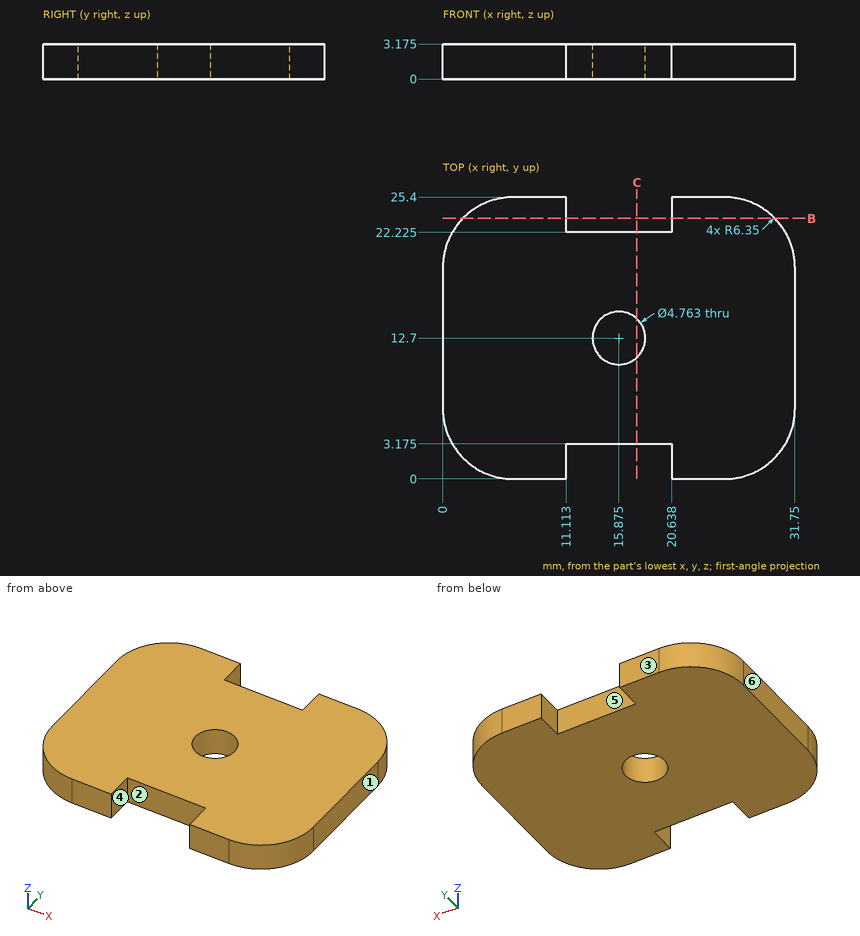
For this review, use the dimensioned drawing (mm, ordinates from the lowest corner) and the shaded views. A direction names the side the tool comes from. Coordinates: 2 decimals unless noted, no trailing zeros. Order: outer loops, then holes, each group sorted by start corner. A loop starts at its lowest first (then second) coordinate and runs counter-clockwise, first axis right, second up. Notation, with made-up numbers: (51, 45) - (67, 45) arc R18 ccw to (67, 50) - close; hole circle Ø1 at (-8, -29). An arc over 180 degrees is marked (long way). Answer in a Markdown table with one row per item.
(1) Consider section C-C on x = 17.5. State the section outline as (y, z) points (1 decimal).
Checked values:
| item | result |
|---|---|
| outline | (3.2, 0) - (11, 0) - (11, 3.2) - (3.2, 3.2) - close; (14.4, 0) - (22.2, 0) - (22.2, 3.2) - (14.4, 3.2) - close |
(2) Clearance check with flat-ended pins moving along their axes: pin 1 (1 mm diameter, centred on y = 1, z = 2, fed in from -X); pin 2 (7.5 mm diameter, centred on x = 15.875, y = 12.7, fed in from -Z); pin 3 (1.6 mm diameter, centred on y = 23, z = 2, fed in from +X) (1 decimal); pin 4 (1 mm diameter, centred on x = 16, z = 2, fed in from +Y) (1 decimal). State where each tip first meets the part, or that it passes through.
Checked values:
| item | result |
|---|---|
| pin 1 | x = 2.25 |
| pin 2 | z = 0 |
| pin 3 | x = 30.9 |
| pin 4 | y = 22.2 |
(3) Consider section B-B on y = 23.5. State the section outline as (x, z) points (1 decimal).
Checked values:
| item | result |
|---|---|
| outline | (1.8, 0) - (11.1, 0) - (11.1, 3.2) - (1.8, 3.2) - close; (20.6, 0) - (29.9, 0) - (29.9, 3.2) - (20.6, 3.2) - close |
(4) The part is to be moulded in two halves that separate along X. For the marked faces 1, 2 and 3, say which applies: released by +X, released by -X, zero draft, split by the parting line, or undercut.
Checked values:
| item | result |
|---|---|
| face 1 | released by +X |
| face 2 | undercut |
| face 3 | zero draft |
(5) For the marked faces 4, 5 and 6, list the 3-axis set-ups (+Z, -Z, +X, -X, +Y, -Y) from which the entire face can be reached by the end or side of a thin tool; tool diameter is ignored.
Checked values:
| item | result |
|---|---|
| face 4 | +Z, -Z, -Y |
| face 5 | +Z, -Z, +Y |
| face 6 | +Z, -Z, -X, +Y, -Y |
(6) Wall thickness on line 1 along Y through (x, z) = (15, 1.95) (1 decimal); line 2 along Y through (x, z) = (12.5, 0.75) (1 decimal); line 3 along Y through (x, z) = (14.5, 1.75) (1 decimal): over which ranges is each line inside the solid? List them lowest first. Write a range as from..to.
Checked values:
| item | result |
|---|---|
| line 1 | 3.2..10.5, 14.9..22.2 |
| line 2 | 3.2..22.2 |
| line 3 | 3.2..10.8, 14.6..22.2 |
